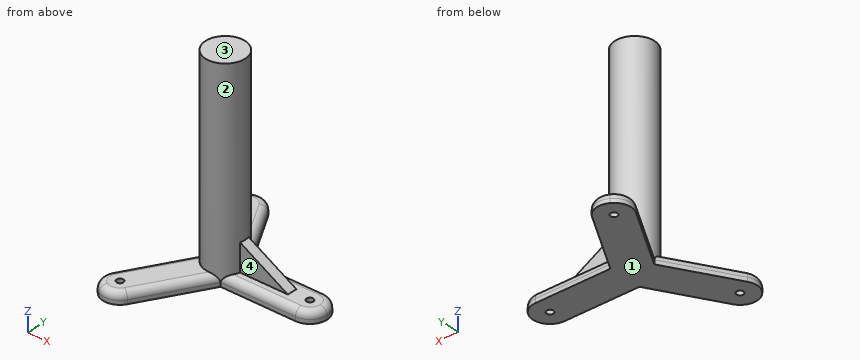
```python
from build123d import *

# Parameters (mm, degrees)
F0_R     = 2.5
F1_DEPTH = 8
F2_R     = 5
F3_R     = 14.5
F4_DEPTH = 140
F5_DEPTH = 8
F7_DEPTH = 20
F9_DEPTH = 80.7


with BuildPart() as f1:
    # F0 (on Top) → F1 (new body)
    with BuildSketch(Plane.XY):
        with BuildLine():
            ThreePointArc((75, 0), (71.3388347648, 8.8388347648), (62.5, 12.5))
            Line((62.5, 12.5), (7.2168783649, 12.5))
            Line((7.2168783649, 12.5), (-20.4246824527, 60.3765877365))
            ThreePointArc((-20.4246824527, 60.3765877365), (-28.0147619362, 66.2006605651), (-37.5, 64.9519052838))
            ThreePointArc((-37.5, 64.9519052838), (-43.3240728286, 57.3618258003), (-42.0753175473, 47.8765877365))
            Line((-42.0753175473, 47.8765877365), (-14.4337567297, 0))
            Line((-14.4337567297, 0), (-42.0753175473, -47.8765877365))
            ThreePointArc((-42.0753175473, -47.8765877365), (-43.3240728286, -57.3618258003), (-37.5, -64.9519052838))
            ThreePointArc((-37.5, -64.9519052838), (-28.0147619362, -66.2006605651), (-20.4246824527, -60.3765877365))
            Line((-20.4246824527, -60.3765877365), (7.2168783649, -12.5))
            Line((7.2168783649, -12.5), (62.5, -12.5))
            ThreePointArc((62.5, -12.5), (71.3388347648, -8.8388347648), (75, 0))
        make_face()
        with Locations((-31.25, -54.1265877365)):
            Circle(F0_R, mode=Mode.SUBTRACT)
        with Locations((62.5, 0)):
            Circle(F0_R, mode=Mode.SUBTRACT)
        with Locations((-31.25, 54.1265877365)):
            Circle(F0_R, mode=Mode.SUBTRACT)
    extrude(amount=F1_DEPTH)

    # F2
    f2_edges = [f1.edges().sort_by_distance(p)[0] for p in [
        (-37.5, 64.951905, 8),
        (-28.254537, -23.938294, 8),
        (34.858439, -12.5, 8),
    ]]
    fillet(f2_edges, radius=F2_R)

    # F3 (on face) → F4 (join)
    with BuildSketch(Plane.XY.offset(8)):
        Circle(F3_R)
    extrude(amount=F4_DEPTH)

    # F5 (add): faces of the model
    f5_faces = [f1.faces().sort_by_distance(p)[0] for p in [
        (6.0657037569, -10.5061070906, 8),
        (6.0657037569, 10.5061070906, 8),
        (-12.1314075138, 0, 8),
    ]]
    extrude(f5_faces, amount=F5_DEPTH)

    # F6 (on face) → F7 (join)
    with BuildSketch(Plane.XY.offset(8)):
        with BuildLine():
            Line((14.024142154, -3.6842145491), (49.3441671133, -3.6842145491))
            Line((49.3441671133, -3.6842145491), (49.3441671133, 3.6842145491))
            Line((49.3441671133, 3.6842145491), (14.024142154, 3.6842145491))
            ThreePointArc((14.024142154, 3.6842145491), (14.3805434743, 1.8574093204), (14.5, 0))
            ThreePointArc((14.5, 0), (14.3805434743, -1.8574093204), (14.024142154, -3.6842145491))
        make_face()
    extrude(amount=F7_DEPTH)

    # F8 (on face) → F9 (cut)
    with BuildSketch(Plane.XZ.offset(3.6842145491)):
        Polygon((14.024142154, 28), (49.3441671133, 8), (49.3441671133, 28), align=None)
    extrude(amount=-F9_DEPTH, mode=Mode.SUBTRACT)


solid = f1.part
```
Design review of the part built by this model. Coordinates are the model's own, in mm. Face numbers are marked on the shaded views. A direction names the side the tool comes from. Coordinates: 2 decimals unless noted, no trailing zeros. Loops run counter-clockwise (first coordinate to the right, second up) from the corner with the lowest first, then second, coordinate; pieces in that order, holes last. Notation, with made-up numbers: (-8.5, -37.75) - (19.5, -37.75) arc R14 cw to (19.5, -24.75) - close; hole circle Ø2 at (75, 28). An arc over 180 degrees is marked (long way). Use CSV: the item, a comma, the result in double quotes. Start each with the question number.
1) Consider section C-C on x = -31.25. Give the number of separate pieces and of enclosed holes in the cut face, then the cut area to 3 significant figures.
2) Consider section B-B on z = 71.5. Write out the cut boundary in (x, y).
3) Consider section A-A on x = 28. Write out the cut boundary in (y, z).
4) Tool access review of the marked faces 1 and 2: name each direction out of +Z, -Z, +X, -X, +Y, -Y from which nothing blocks a thin tool from reaching the whole face with its end or side.
5) The part is to be moulded in two halves that separate along Y. For the marked faces 3 and 4, say which applies: +Y half, -Y half, draft (parallel to the pull), parting line (faces both ways), or undercut.
6) For pin 1 Ø1.5 at (x, z) = (21, 21) entering from +Y; pin 2 Ø0.9 at (x, z) = (40.5, 1) entering from -Y; pin 3 Ø1.5 at (y, z) = (16, 119) entering from +X; pin 4 Ø6 at (x, z) = (-12.5, 113) entering from -Y, all flat-tipped, find the tip position at first contact; note any pin that passes through.
7) Consider section D-D on z = 23. Write out the cut boundary in (x, y), then the cut area to 3 significant figures.
8) Wall thickness on L1, parallel to Y at x = -31.25, z = 6.75; L2, parallel to Y at x = -31, z = 5; L3, parallel to Z at x = 37.5, y = 7.5: over which ranges is each line inside the solid? List them lowest first. Write a range as from..to.
Geometry says:
1,separate pieces,"4"
1,enclosed holes,"0"
1,area,"488 mm^2"
2,outline,"circle Ø29 at (0, 0)"
3,outline,"(-12.5, 0) - (12.5, 0) - (12.5, 3) arc R5 ccw to (7.5, 8) - (3.68, 8) - (3.68, 20.09) - (-3.68, 20.09) - (-3.68, 8) - (-7.5, 8) arc R5 ccw to (-12.5, 3) - close"
4,face 1,"-Z, +X, -X, +Y, -Y"
4,face 2,"+Z"
5,face 3,"draft"
5,face 4,"-Y half"
6,pin 1,"y = 3.68"
6,pin 2,"y = -12.5"
6,pin 3,"through"
6,pin 4,"y = -10.95"
7,outline,"(14.02, -3.68) - (22.85, -3.68) - (22.85, 3.68) - (14.02, 3.68) arc R14.5 ccw (long way) to start"
7,area,"723 mm^2"
8,L1,"-64.93..-56.63, -51.63..-32.51, 32.51..51.63, 56.63..64.93"
8,L2,"-66.21..-56.61, -51.64..-29.53, 29.53..51.64, 56.61..66.21"
8,L3,"0..8"
